Autodesk Inventor part; units mm, degrees
ref_plane "YZ Plane" through (0, 0, 0) normal (1, 0, 0) x (0, 1, 0)
ref_plane "XZ Plane" through (0, 0, 0) normal (0, 1, 0) x (-1, 0, 0)
ref_plane "XY Plane" through (0, 0, 0) normal (0, 0, 1) x (1, 0, 0)
sketch "スケッチ1" plane through (0, 0, 0) normal (0, 1, 0) x (-1, 0, 0)
  line L0 (0, 0) -> (-9, 0)
  line L1 (-9, 0) -> (-9, 9)
  line L2 (-9, 9) -> (0, 9)
  line L3 (0, 9) -> (0, 0)
  line L4 (-1.2, 7.8) -> (-7.8, 7.8)
  line L5 (-7.8, 7.8) -> (-7.8, 1.2)
  line L6 (-7.8, 1.2) -> (-1.2, 1.2)
  line L7 (-1.2, 1.2) -> (-1.2, 7.8)
  dimension "d0" = 9
  dimension "d1" = 9
  dimension "d2" = 1.2
  dimension "d3" = 1.2
  dimension "d4" = 1.2
  dimension "d5" = 1.2
extrude "押し出し1" add sketch "スケッチ1" along normal blind 92.5
sketch "スケッチ2" plane through (9, 0, 9) normal (1, 0, 0) x (0, 0, -1)
  line L0 (0, 0) -> (9, 0)
  line L1 (0, 0) -> (0, 92.5)
  point P0 (4.5, 5)
  point P1 (4.5, 35)
  dimension "d8" = 30
  dimension "d9" = 5
  dimension "d10" = 4.5
  dimension "d11" = 4.5
hole "穴1" at (9, 5, 4.5) at (9, 35, 4.5) direction (-1, 0, 0) diameter 3.3 end through all
sketch "スケッチ5" plane through (9, 0, 0) normal (0, 0, -1) x (-1, 0, 0)
  line L0 (0, 92.5) -> (9, 92.5)
  line L1 (9, 0) -> (9, 92.5)
  point P0 (4.5, 79)
  dimension "d41" = 13.5
  dimension "d42" = 4.5
hole "穴4" at (4.5, 79, 0) direction (0, 0, 1) diameter 3 end through all
sketch "スケッチ6" plane through (0, 0, 0) normal (-1, 0, 0) x (0, 0, 1)
  line L0 (0, 92.5) -> (9, 92.5)
  line L1 (0, 0) -> (0, 92.5)
  point P0 (4.5, 88)
  dimension "d50" = 4.5
  dimension "d51" = 4.5
hole "穴5" at (0, 88, 4.5) direction (1, 0, 0) diameter 3 end through all
sketch "スケッチ7" plane through (0, 0, 9) normal (0, 0, 1) x (1, 0, 0)
  circle A0 centre (4.5, 79) radius 1.5
  line L0 (0, 0) -> (0, 92.5)
  point P0 (4.5, 73)
  point P1 (4.5, 67)
  point P2 (4.5, 61)
  point P3 (4.5, 55)
  point P4 (4.5, 49)
  point P5 (4.5, 43)
  point P6 (4.5, 37)
  point P7 (4.5, 31)
  point P8 (4.5, 25)
  point P9 (4.5, 19)
  point P10 (4.5, 13)
  point P11 (4.5, 7)
  dimension "d59" = 6
  dimension "d60" = 4.5
  dimension "d63" = 6
  dimension "d70" = 6
  dimension "d77" = 6
hole "穴6" at (4.5, 73, 9) at (4.5, 67, 9) at (4.5, 61, 9) at (4.5, 55, 9) at (4.5, 49, 9) at (4.5, 43, 9) at (4.5, 37, 9) at (4.5, 31, 9) at (4.5, 25, 9) at (4.5, 19, 9) at (4.5, 13, 9) at (4.5, 7, 9) direction (0, 0, -1) diameter 4 end through all
sketch "スケッチ8" plane through (9, 0, 9) normal (1, 0, 0) x (0, 0, -1)
  line L0 (0, 0) -> (0, 92.5)
  circle A0 centre (4.5, 5) radius 1.65
  point P0 (9, 0)
  point P1 (4.5, 9.5)
  point P2 (4.5, 14.5)
  point P3 (4.5, 19.5)
  point P4 (4.5, 24.5)
  point P5 (4.5, 29.5)
  dimension "d89" = 4.5
  dimension "d90" = 4.5
  dimension "d93" = 5
hole "穴7" at (9, 9.5, 4.5) at (9, 14.5, 4.5) at (9, 19.5, 4.5) at (9, 24.5, 4.5) at (9, 29.5, 4.5) direction (-1, 0, 0) diameter 4 end through all
sketch "スケッチ9" plane through (9, 0, 9) normal (1, 0, 0) x (0, 0, -1)
  line L0 (0, 0) -> (0, 92.5)
  circle A0 centre (4.5, 88) radius 1.5
  point P0 (9, 0)
  point P1 (4.5, 83)
  point P2 (4.5, 77.8)
  point P3 (4.5, 72.6)
  point P4 (4.5, 67.4)
  point P5 (4.5, 62.2)
  point P6 (4.5, 57)
  point P7 (4.5, 51.8)
  point P8 (4.5, 46.6)
  point P9 (4.5, 41.4)
  dimension "d105" = 4.5
  dimension "d106" = 5
  dimension "d109" = 5.2
hole "穴8" at (9, 83, 4.5) at (9, 77.8, 4.5) at (9, 72.6, 4.5) at (9, 67.4, 4.5) at (9, 62.2, 4.5) at (9, 57, 4.5) at (9, 51.8, 4.5) at (9, 46.6, 4.5) at (9, 41.4, 4.5) direction (-1, 0, 0) diameter 4 end through all
sketch "スケッチ10" plane through (0, 0, 9) normal (0, 0, 1) x (1, 0, 0)
  line L0 (9, 0) -> (9, 92.5)
  line L1 (0, 92.5) -> (9, 92.5)
  point P0 (0, 0)
  point P1 (4.5, 85.75)
  dimension "d121" = 4.5
  dimension "d122" = 6.75
hole "穴9" at (4.5, 85.75, 9) direction (0, 0, -1) diameter 5 end through all
equation "\"d3\" = d2"
equation "\"d4\" = d2"
equation "\"d5\" = d3"
properties part number "ハンド9x9_1_CPY" material "アルミニウム 6061"
Read the model definition and answer for the solid it produces. Units are mm, in the model's axes. A direction names the side the tool comes from. Round coordinates to 2 decimals unless told otherwise and drop trailing zeros. Loops run counter-clockwise (first coordinate to the right, second up) from the corner with the lowest first, then second, coordinate; pieces in that order, holes last.
Q1. Consider probe 1 along X at (y, z) = (13, 0.6); probe 2 along Z at (x, y) = (1.5, 10). Determine where each line is inside the solid, lowest interval first.
Q2. Section B-B on x = 4.5 is taken. Give the number of separate pieces and of enclosed holes in the cut face, and give its area (3 significant figures).
Q3. Section C-C on y = 72.6 is taken. Write down the section's boundary in (x, z), and give its area (3 significant figures).
Q4. Which of the six approach directions +Z, -Z, +X, -X, +Y, -Y give full straight-line access (tool end or side, diameter ignored) to faces 1 (the face through (5.7, 14.6, 8.4)), 2 (the face through (5, 46, 1.2))?
Q5. Section A-A on y = 62.2 is taken. Write down the section's boundary in (x, z), and give its area (3 significant figures).
Q6. Determine the mould class of faces 3 (the face through (1.2, 46, 2)), 4 (the face through (0.6, 25.7, 6.1)) for opening direction Y: released by +Y, released by -Y, zero draft, split by the parting line, or undercut.
Output:
1. probe 1: x = 0 to 2.5, 6.5 to 9
1. probe 2: z = 0 to 1.2, 7.8 to 9
2. separate pieces: 30
2. enclosed holes: 0
2. area: 87.6 mm2
3. outline: (0, 0) - (2.54, 0) - (2.54, 1.2) - (1.2, 1.2) - (1.2, 2.5) - (0, 2.5) - close; (0, 6.5) - (1.2, 6.5) - (1.2, 7.8) - (2.54, 7.8) - (2.54, 9) - (0, 9) - close; (6.46, 0) - (9, 0) - (9, 2.5) - (7.8, 2.5) - (7.8, 1.2) - (6.46, 1.2) - close; (6.46, 7.8) - (7.8, 7.8) - (7.8, 6.5) - (9, 6.5) - (9, 9) - (6.46, 9) - close
3. area: 18.4 mm2
4. face 1: +Z, -Z
4. face 2: +Y, -Y
5. outline: (0, 0) - (2.9, 0) - (2.9, 1.2) - (1.2, 1.2) - (1.2, 2.5) - (0, 2.5) - close; (0, 6.5) - (1.2, 6.5) - (1.2, 7.8) - (2.9, 7.8) - (2.9, 9) - (0, 9) - close; (6.1, 0) - (9, 0) - (9, 2.5) - (7.8, 2.5) - (7.8, 1.2) - (6.1, 1.2) - close; (6.1, 7.8) - (7.8, 7.8) - (7.8, 6.5) - (9, 6.5) - (9, 9) - (6.1, 9) - close
5. area: 20.2 mm2
6. face 3: zero draft
6. face 4: undercut
